Design review of the part shown in the three views and the two pictorial views. Dimensions are in mm from the part's minimum x, y and z. Coordinates: 2 decimals unless noted, no trailing zeros. Order: outer loops, then holes, each group sorted by start corner. A loop starts at its lowest first (then second) coordinate and runs counter-clockwise, first axis right, second up. Notation, with made-up numbers: M 38,42.25 L 42,42.25 A7 cw 42,46.25 Z; hole C 83.5,37.25 d11. An arc over 180 degrees is marked long. Use CSV: the item, a comma, the result in double quotes.
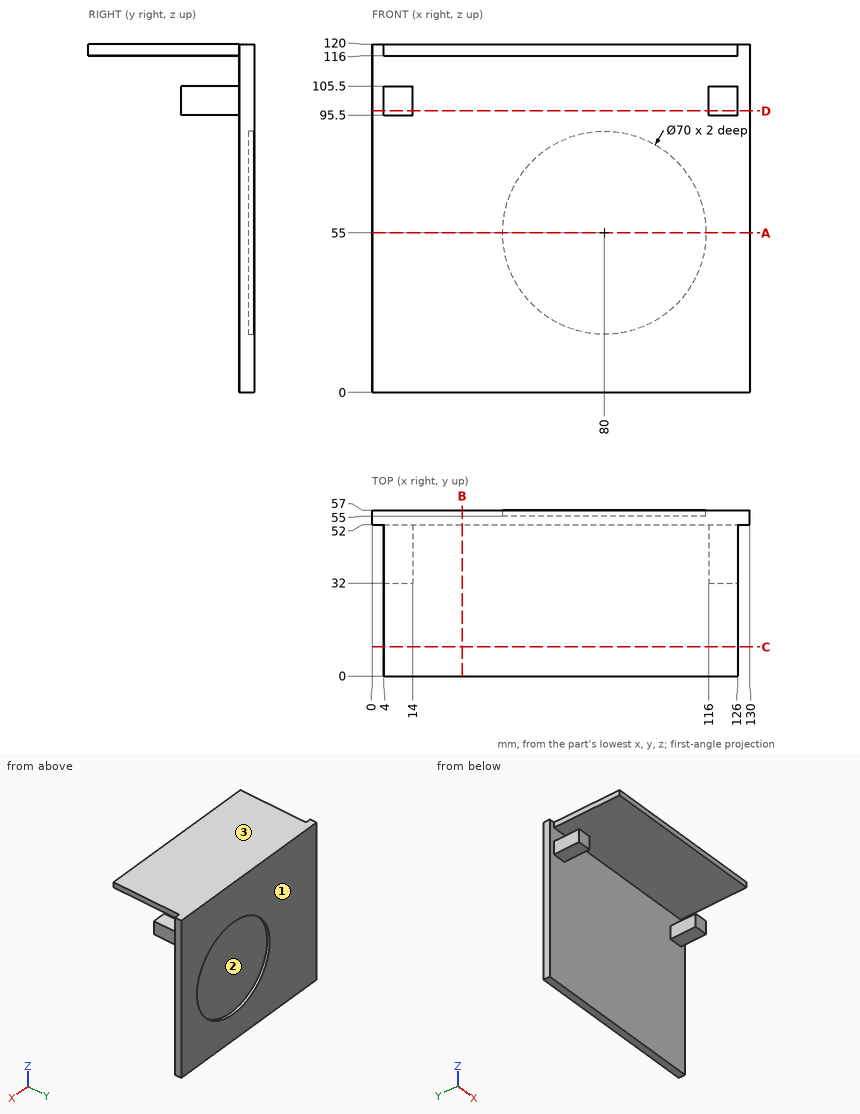
(1) Wall thickness on probe 1 along X at (y, z) = (56, 55); probe 2 along Y at (x, z) = (6, 14); probe 3 along Z at (x, y) = (102, 27): over which ranges is each line inside the solid? List them lowest first.
The answers:
probe 1,"x = 0 to 45, 115 to 130"
probe 2,"y = 52 to 57"
probe 3,"z = 116 to 120"
(2) Add section D-D on z = 97. State the section outline as (x, y) points.
The answers:
outline,"M 0,52 L 4,52 L 4,32 L 14,32 L 14,52 L 116,52 L 116,32 L 126,32 L 126,52 L 130,52 L 130,57 L 0,57 Z"
(3) Add section C-C on y = 10. State the section outline as (x, z) points.
The answers:
outline,"M 4,116 L 126,116 L 126,120 L 4,120 Z"
(4) Add section A-A on z = 55. State the section outline as (x, y) points, and give its area (3 significant figures).
The answers:
outline,"M 0,52 L 130,52 L 130,57 L 115,57 L 115,55 L 45,55 L 45,57 L 0,57 Z"
area,"510 mm2"
(5) Add section B-B on x = 31. State the section outline as (y, z) points.
The answers:
outline,"M 0,116 L 52,116 L 52,0 L 57,0 L 57,120 L 0,120 Z"
(6) The part is to be moulded in two halves that separate along Z. For the marked faces 1, 2 and 3, say which applies: pulls with the +Z half, pulls with the -Z half, needs draft (parallel to the pull), parting line crosses it, or undercut.
The answers:
face 1,"needs draft"
face 2,"undercut"
face 3,"pulls with the +Z half"
(7) Clearance check with flat-ended pins moving along their axes: P1, Ø21, axis at x = 87, z = 60.5, coming from the +Y side; P2, Ø2, axis at y = 36, z = 118, coming from the +X side; P3, Ø11, axis at y = 40, z = 100.5, coming from the -X side. State where each tip first meets the part, or that it passes through.
The answers:
P1,"stops at y = 55"
P2,"stops at x = 126"
P3,"stops at x = 4"
